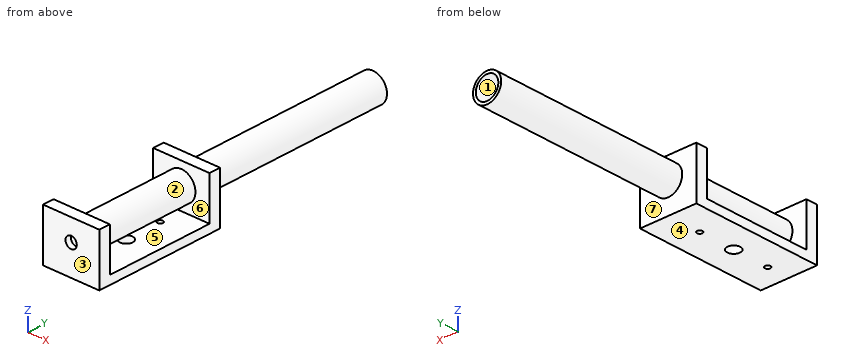
```python
from build123d import *

# Parameters (mm, degrees)
SKETCH1_W           = 20
SKETCH1_H           = 46
SKETCH1_R           = 0.955
SKETCH1_R_2         = 2.3
BOSS_EXTRUDE1_DEPTH = 3
SKETCH2_W           = 20
SKETCH2_H           = 15
SKETCH2_R           = 4
BOSS_EXTRUDE2_DEPTH = 4
SKETCH4_R           = 5
SKETCH4_R_2         = 4
BOSS_EXTRUDE4_DEPTH = 115
SKETCH5_W           = 20
SKETCH5_H           = 15
SKETCH5_R           = 4
BOSS_EXTRUDE6_DEPTH = 4
SKETCH4_3_R         = 3.25
SKETCH4_3_R_2       = 2
BOSS_EXTRUDE7_DEPTH = 2
SKETCH4_4_R         = 4
SKETCH4_4_R_2       = 3.25
BOSS_EXTRUDE8_DEPTH = 3


with BuildPart() as part:
    # Sketch1 → Boss-Extrude1 (new body)
    with BuildSketch(Plane.XY):
        with Locations((11.641947403, 2)):
            Rectangle(SKETCH1_W, SKETCH1_H)
        with Locations((11.599686328, 13)):
            Circle(SKETCH1_R, mode=Mode.SUBTRACT)
        with Locations((11.684208477, -13)):
            Circle(SKETCH1_R, mode=Mode.SUBTRACT)
        with Locations((11.641947403, 0)):
            Circle(SKETCH1_R_2, mode=Mode.SUBTRACT)
    extrude(amount=BOSS_EXTRUDE1_DEPTH)

    # Sketch2 → Boss-Extrude2 (add)
    with BuildSketch(Plane.XZ.offset(21)):
        with Locations((11.641947403, 10.5)):
            Rectangle(SKETCH2_W, SKETCH2_H)
        with Locations((11.641947403, 10.5)):
            Circle(SKETCH2_R, mode=Mode.SUBTRACT)
    extrude(amount=-BOSS_EXTRUDE2_DEPTH)

    # Sketch4 → Boss-Extrude4 (add)
    with BuildSketch(Plane.XZ.offset(21)):
        with Locations((11.641947403, 10.5)):
            Circle(SKETCH4_R)
        with Locations((11.641947403, 10.5)):
            Circle(SKETCH4_R_2, mode=Mode.SUBTRACT)
    extrude(amount=-BOSS_EXTRUDE4_DEPTH)

    # Sketch5 → Boss-Extrude6 (add)
    with BuildSketch(Plane(origin=(0, 25, 0), x_dir=(1, 0, 0), z_dir=(0, 1, 0))):
        with Locations((11.641947403, -10.5)):
            Rectangle(SKETCH5_W, SKETCH5_H)
        with Locations((11.641947403, -10.5)):
            Circle(SKETCH5_R, mode=Mode.SUBTRACT)
    extrude(amount=-BOSS_EXTRUDE6_DEPTH)



with BuildPart() as body_2:
    # Sketch4_3 → Boss-Extrude7 (new body)
    with BuildSketch(Plane.XZ.offset(21)):
        with Locations((11.641947403, 10.5)):
            Circle(SKETCH4_3_R)
        with Locations((11.641947403, 10.5)):
            Circle(SKETCH4_3_R_2, mode=Mode.SUBTRACT)
    extrude(amount=-BOSS_EXTRUDE7_DEPTH)


with BuildPart() as part_1:
    add(part.part)

    add(body_2.part)  # Boss-Extrude8 merges body 2
    # Sketch4_4 → Boss-Extrude8 (add)
    with BuildSketch(Plane.XZ.offset(21)):
        with Locations((11.641947403, 10.5)):
            Circle(SKETCH4_4_R)
        with Locations((11.641947403, 10.5)):
            Circle(SKETCH4_4_R_2, mode=Mode.SUBTRACT)
    extrude(amount=-BOSS_EXTRUDE8_DEPTH)


solid = part_1.part
```
CAD build for the part. Positions are in the model's coordinates, mm. Face numbers are marked on the shaded views. A direction names the side the tool comes from. Coordinates: 2 decimals unless noted, no trailing zeros. Order: outer loops, then holes, each group sorted by start corner. A loop starts at its lowest first (then second) coordinate and runs counter-clockwise, first axis right, second up. Notation, with made-up numbers: M 37.5,-8 L 44.5,-8 A17 ccw 44.5,12 Z; hole C 37.5,3.5 d10. An arc over 180 degrees is marked long. Write each question's results on one line, items separated by ' | '. Start each with the question number.
Q1. Cut at D-D (z = 1.5). List the corners of the cut face in (x, y) (3 decimals), then the cut area to 3 significant figures.
Q2. Cut at A-A (y = 13). List the corners of the cut face in (x, z).
Q3. Drill centre lines: probe 1 along Y at (x, z) = (11.75, 1.25); probe 2 along Y at (x, z) = (6.25, 14.5); probe 3 along Z at (x, y) = (9.25, 18.5). Where is each one in solid material? Low to high. Write a range as from..to.
Q4. Cut at B-B (z = 10.5). List the corners of the cut face in (x, y), then the cut area to 4 significant figures.
Q5. Flat gauge pins, fed straight in: P1, Ø1.5, axis at y = 41, z = 15, coming from the +X side; P2, Ø10, axis at y = 56.5, z = 2.5, coming from the -X side; P3, Ø1, axis at y = 47.5, z = 6.5, coming from the +X side. Where does each tip first touch, or does it go through?
Q6. Cut at C-C (y = -6.5). List the corners of the cut face in (x, z), then the cut area to 3 significant figures.
Q7. Which spindle directions (+Z, -Z, +X, -X, +Y, -Y) get a long thin tool onto all of the face, cutting with end or side? Do the marked faces 4, 5, 6 and 7. Say none if no direction does.
Q8. Pull direction X, two halves, no side cores. Call the marked faces 1, 2 and 3: +X half, -X half, draft (parallel to the pull), parting line (faces both ways), or undercut.
Found:
1) outline: M 1.642,-21 L 21.642,-21 L 21.642,25 L 1.642,25 Z; hole C 11.642,0 d4.6; hole C 11.6,13 d1.91; hole C 11.684,-13 d1.91 | area: 898 mm²
2) outline: M 1.64,0 L 10.64,0 L 10.64,3 L 1.64,3 Z; C 11.64,10.5 d10; M 12.55,0 L 21.64,0 L 21.64,3 L 12.55,3 Z; hole C 11.64,10.5 d8
3) probe 1: -21..-13.95, -12.05..-2.3, 2.3..12.06, 13.94..25 | probe 2: -21..-17, 21..25 | probe 3: 0..3, 6.11..7.29, 13.71..14.89
4) outline: M 1.64,-21 L 9.64,-21 L 9.64,-19 L 8.39,-19 L 8.39,-18 L 7.64,-18 L 7.64,94 L 6.64,94 L 6.64,25 L 1.64,25 L 1.64,21 L 6.64,21 L 6.64,-17 L 1.64,-17 Z; M 13.64,-21 L 21.64,-21 L 21.64,-17 L 16.64,-17 L 16.64,21 L 21.64,21 L 21.64,25 L 16.64,25 L 16.64,94 L 15.64,94 L 15.64,-18 L 14.89,-18 L 14.89,-19 L 13.64,-19 Z | area: 319.5 mm²
5) P1: x = 14.95 | P2: x = 7.64 | P3: x = 15.21
6) outline: M 1.64,0 L 21.64,0 L 21.64,3 L 1.64,3 Z; C 11.64,10.5 d10; hole C 11.64,10.5 d8 | area: 88.3 mm²
7) face 4: -Z, +X, -X, +Y, -Y | face 5: +X, -X | face 6: none | face 7: +Y
8) face 1: undercut | face 2: parting line | face 3: draft
